Autodesk Inventor part; units mm, degrees
ref_plane "YZ Plane" through (0, 0, 0) normal (1, 0, 0) x (0, 1, 0)
ref_plane "XZ Plane" through (0, 0, 0) normal (0, 1, 0) x (-1, 0, 0)
ref_plane "XY Plane" through (0, 0, 0) normal (0, 0, 1) x (1, 0, 0)
sketch "Sketch1" plane through (0, 0, 0) normal (0, 1, 0) x (-1, 0, 0)
  line L0 (0, 0) -> (23.5, 0)
  line L1 (23.5, 0) -> (23.5, -23.5)
  line L2 (23.5, -23.5) -> (0, -23.5)
  line L3 (0, -23.5) -> (0, 0)
  dimension "d0" = 23.5
  dimension "d1" = 23.5
extrude "Extrusion1" add sketch "Sketch1" along normal blind 8
sketch "Sketch2" plane through (0, 0, 0) normal (1, 0, 0) x (0, 0, -1)
  circle A0 centre (4, 4) radius 2
  circle A1 centre (12, 4) radius 2
  circle A2 centre (20, 4) radius 2
  line L0 (0, 0) -> (0, 8)
  point P0 (0, 4)
  dimension "d4" = 4
  dimension "d5" = 4
  dimension "d6" = 4
  dimension "d7" = 4
  dimension "d8" = 8
  dimension "d9" = 8
extrude "Extrusion2" add sketch "Sketch2" along normal blind 2
sketch "Sketch3" plane through (-23.5, 0, 0) normal (0, 0, 1) x (1, 0, 0)
  circle A0 centre (19.5, 4) radius 2.175
  circle A1 centre (11.5, 4) radius 2.175
  circle A2 centre (3.5, 4) radius 2.175
  line L0 (23.5, 0) -> (23.5, 8)
  dimension "d12" = 4.35
  dimension "d13" = 4.35
  dimension "d14" = 4.35
  dimension "d15" = 4
  dimension "d16" = 8
  dimension "d17" = 8
extrude "Extrusion3" cut sketch "Sketch3" against normal blind 27
sketch "Sketch6" plane through (0, 0, 0) normal (0, -1, 0) x (1, 0, 0)
  line L0 (-23.5, 0) -> (0, 0)
  line L1 (0, -23.5) -> (-23.5, -23.5)
  line L2 (-23.5, 0) -> (0, 0)
  line L3 (0, 0) -> (0, -23.5)
  line L4 (0, -23.5) -> (-23.5, -23.5)
  line L5 (-23.5, -23.5) -> (-23.5, 0)
extrude "Extrusion5" add sketch "Sketch6" along normal blind 4.5
fillet "Fillet1" radius 4.5 4 edges at (-11.75, -4.5, 0) (0, -4.5, -11.75) (-11.75, -4.5, -23.5) (-23.5, -4.5, -11.75)
fillet "Fillet2" radius 1 8 edges at (-1.318, -3.182, -1.318) (0, 4, 0) (-1.318, -3.182, -22.182) (0, 4, -23.5) (-23.5, 4, -23.5) (-22.182, -3.182, -22.182) (-23.5, 4, 0) (-22.182, -3.182, -1.318)
properties part number "base_support"
Read the model definition and answer for the solid it produces. Units are mm, in the model's axes. A direction names the side the tool comes from. Coordinates: 2 decimals unless noted, no trailing zeros. Loops run counter-clockwise (first coordinate to the right, second up) from the corner with the lowest first, then second, coordinate; pieces in that order, holes last.
(1) The part is cut by section A-A (x = -12). Determine the outline of the cut face in (y, z) (3 decimals).
Solution:
outline: (-4.5, -19) arc R4.5 ccw to (0, -23.5) - (1.825, -23.5) - (1.825, 0) - (0, 0) arc R4.5 ccw to (-4.5, -4.5) - close; (6.175, -23.5) - (8, -23.5) - (8, 0) - (6.175, 0) - close
(2) A tool of negligible diameter and unlimited length cuts with its end or side. For faces 1 (the face through (-9.925, 4.653, -11.586)), 2 (the face through (1, 5.2, -10.4)), from which of +Z, -Z, +X, -X, +Y, -Y can it reach the whole face along a straight path? Write none if from no direction.
Solution:
face 1: +Z, -Z
face 2: +X
(3) The part is cut by section D-D (z = -12). Determine the outline of the cut face in (x, y) (3 decimals).
Solution:
outline: (-23.5, 0) arc R4.5 ccw to (-19, -4.5) - (-4.5, -4.5) arc R4.5 ccw to (0, 0) - (0, 2) - (2, 2) - (2, 6) - (0, 6) - (0, 8) - (-23.5, 8) - close; hole circle Ø4.35 at (-20, 4); hole circle Ø4.35 at (-12, 4); hole circle Ø4.35 at (-4, 4)
(4) Consider line 1 along Y through (x, z) = (-12, -16.5) (3 decimals); line 2 along X through (y, z) = (3.75, -21); line 3 along X through (y, z) = (3.5, -17.5). Determine where each line is inside the solid, lowest interval first.
Solution:
line 1: y = -4.5 to 1.825, 6.175 to 8
line 2: x = -23.5 to -22.16, -17.84 to -14.16, -9.84 to -6.16, -1.84 to 2
line 3: x = -23.5 to -22.12, -17.88 to -14.12, -9.88 to -6.12, -1.88 to 0
(5) A flat-ended cylindrical pin translates along its axis: pin 1 Ø1 at (x, y) = (-3, 3) entering from -Z. Find the tip coordinate at first contact, or state that the pin passes through.
Solution:
pin 1: passes through
(6) The part is cut by section B-B (z = -16.25). Determine the outline of the cut face in (x, y) (3 decimals).
Solution:
outline: (-23.5, 0) arc R4.5 ccw to (-19, -4.5) - (-4.5, -4.5) arc R4.5 ccw to (0, 0) - (0, 8) - (-23.5, 8) - close; hole circle Ø4.35 at (-20, 4); hole circle Ø4.35 at (-12, 4); hole circle Ø4.35 at (-4, 4)
(7) The mould has two halves that part along X. Classify faces 3 (the face through (-0.301, 3.944, -23.215)), 4 (the face through (-1.925, 4.653, -11.586)), 5 (the face through (-9.5, 4.1, 0)): released by +X, released by -X, zero draft, split by the parting line, or undercut.
Solution:
face 3: released by +X
face 4: undercut
face 5: zero draft
(8) The part is cut by section C-C (y = 4). Count the separate pieces of the cut face and the enclosed holes in it, and give its area (3 significant figures).
Solution:
separate pieces: 4
enclosed holes: 0
area: 269 mm2
